from build123d import *

# Parameters (mm, degrees)
F1_DEPTH  = 9.5
F2_R      = 3
F3_DEPTH  = 8
F4_R      = 1.75
F5_DEPTH  = 17
F6_W      = 16
F6_H      = 16
F6_W_2    = 15
F6_H_2    = 15
F7_DEPTH  = 5
F8_R      = 2
F9_R      = 4
F9_R_2    = 1.75
F10_DEPTH = 7.5


with BuildPart() as f1:
    # F0 (on Front) → F1 (new body, symmetric)
    with BuildSketch(Plane.XZ):
        Polygon((-9.5, 0), (0, 0), (9.5, 0), (9.5, 9), (-9.5, 9), align=None)
    extrude(amount=F1_DEPTH, both=True)

    # F2 (on face) → F3 (join)
    with BuildSketch(Plane.XY.offset(9)):
        Circle(F2_R)
    extrude(amount=F3_DEPTH)

    # F4 (on face) → F5 (cut)
    with BuildSketch(Plane.XY.offset(17)):
        Circle(F4_R)
    extrude(amount=-F5_DEPTH, mode=Mode.SUBTRACT)

    # F6 (on face) → F7 (cut)
    with BuildSketch(Plane(origin=(0, 0, 0), x_dir=(1, 0, 0), z_dir=(0, 0, -1))):
        Rectangle(F6_W, F6_H)
        Rectangle(F6_W_2, F6_H_2, mode=Mode.SUBTRACT)
    extrude(amount=-F7_DEPTH, mode=Mode.SUBTRACT)

    # F8
    f8_edges = [f1.edges().sort_by_distance(p)[0] for p in [
        (-9.5, -9.5, 4.5),
        (9.5, -9.5, 4.5),
        (-9.5, 9.5, 4.5),
        (9.5, 9.5, 4.5),
    ]]
    fillet(f8_edges, radius=F8_R)

    # F9 (on face) → F10 (cut)
    with BuildSketch(Plane(origin=(0, 0, 0), x_dir=(1, 0, 0), z_dir=(0, 0, -1))):
        Circle(F9_R)
        Circle(F9_R_2, mode=Mode.SUBTRACT)
    extrude(amount=-F10_DEPTH, mode=Mode.SUBTRACT)


solid = f1.part
Input: part model. Units: mm. Frame: model coordinates. A direction names the side the tool comes from. Round coordinates to 2 decimals unless told otherwise and drop trailing zeros. Order: outer loops, then holes, each group sorted by start corner. A loop starts at its lowest first (then second) coordinate and runs counter-clockwise, first axis right, second up. Notation, with made-up numbers: (14.5, 67.5) - (37.5, 67.5) arc R21 cw to (37.5, 94.5) - close; hole circle Ø11 at (85, 70.25). An arc over 180 degrees is marked (long way). Answer as a JSON object with one key per item and string values. Group by question number.
(1) Pin query (flat end, axial travel): P1, Ø5.5, axis at x = 0, y = 0, coming from the -Z side; P2, Ø4, axis at y = 6, z = 14.5, coming from the -X side. Return the tip coordinate at first contact, or that it passes through.
(2) Cut plane B-B (x = 0). Return loops of the section in (y, z).
(3) Reachability of faces 5 (the face through (-3, 0, 13)), 6 (the face through (-3, -3, 0)), 7 (the face through (0, 8, 2)) from +Z, -Z, +X, -X, +Y, -Y: full face, straight path, thin tool, end or side. Return the list, or none.
(4) Material intervals for probe 1 along Y at (x, z) = (6.75, 3.5); probe 2 along Y at (x, z) = (0, 3.25), sorted ascending. Write a range as from..to.
(5) Cut plane D-D (z = 6.5). Return loops of the section in (x, y).
(6) Cut plane A-A (z = 3). Return loops of the section in (x, y).
(7) Draft query along X for faces 1 (the face through (8.9, 8.93, 4.56)), 2 (the face through (0, -9.5, 5)), 3 (the face through (-8, 0, 2)), 4 (the face through (-8.9, 8.93, 4.44)). Return one class per face: released by +X, released by -X, zero draft, split by the parting line, or undercut.
Here are the results:
{
 "1": {"P1": "stops at z = 7.5", "P2": "passes through"},
 "2": {"outline": "(-9.5, 0) - (-8, 0) - (-8, 5) - (-7.5, 5) - (-7.5, 0) - (-4, 0) - (-4, 7.5) - (-1.75, 7.5) - (-1.75, 17) - (-3, 17) - (-3, 9) - (-9.5, 9) - close; (1.75, 7.5) - (4, 7.5) - (4, 0) - (7.5, 0) - (7.5, 5) - (8, 5) - (8, 0) - (9.5, 0) - (9.5, 9) - (3, 9) - (3, 17) - (1.75, 17) - close"},
 "3": {"face 5": "+Z", "face 6": "-Z, +X, -X, +Y, -Y", "face 7": "-Z"},
 "4": {"probe 1": "y = -9.5..-8, -7.5..7.5, 8..9.5", "probe 2": "y = -9.5..-8, -7.5..-4, 4..7.5, 8..9.5"},
 "5": {"outline": "(-9.5, -7.5) arc R2 ccw to (-7.5, -9.5) - (7.5, -9.5) arc R2 ccw to (9.5, -7.5) - (9.5, 7.5) arc R2 ccw to (7.5, 9.5) - (-7.5, 9.5) arc R2 ccw to (-9.5, 7.5) - close; hole circle Ø8 at (0, 0)"},
 "6": {"outline": "(-9.5, -7.5) arc R2 ccw to (-7.5, -9.5) - (7.5, -9.5) arc R2 ccw to (9.5, -7.5) - (9.5, 7.5) arc R2 ccw to (7.5, 9.5) - (-7.5, 9.5) arc R2 ccw to (-9.5, 7.5) - close; (-7.5, -7.5) - (7.5, -7.5) - (7.5, 7.5) - (-7.5, 7.5) - close; hole (-8, -8) - (8, -8) - (8, 8) - (-8, 8) - close; hole circle Ø8 at (0, 0)"},
 "7": {"face 1": "released by +X", "face 2": "zero draft", "face 3": "undercut", "face 4": "released by -X"}
}
